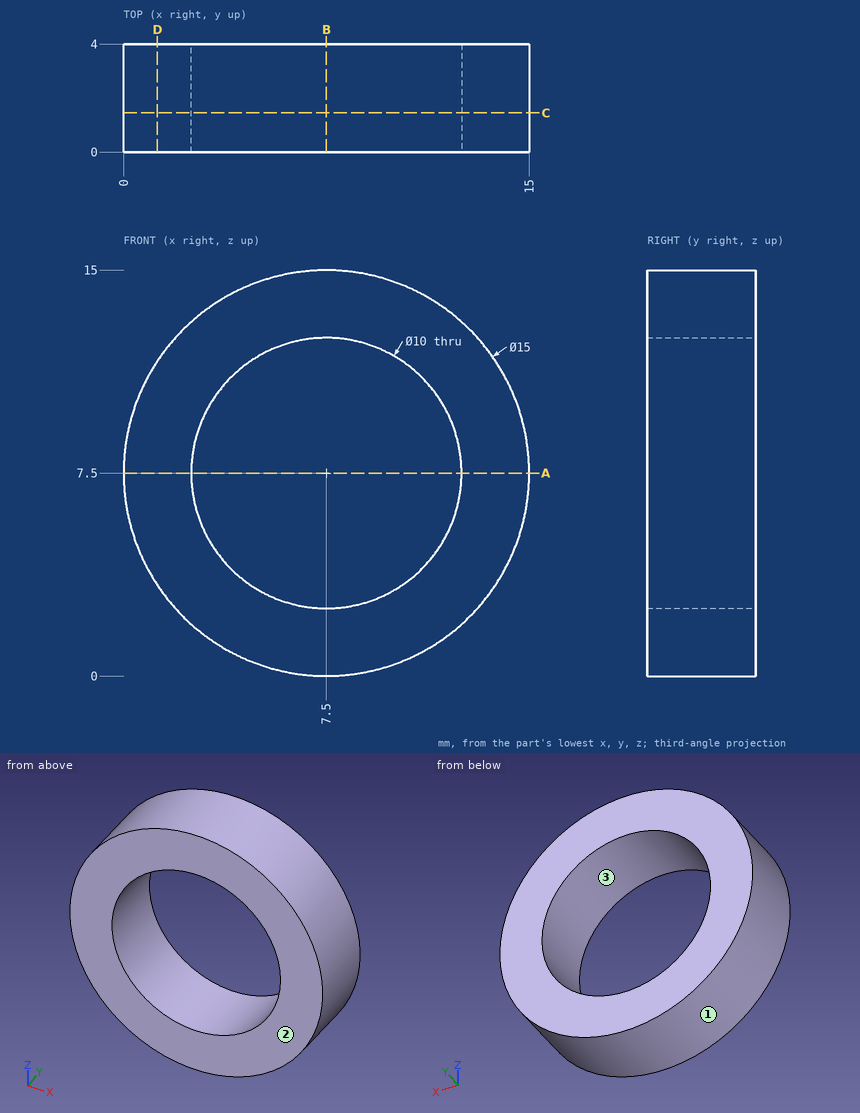
Input: dimensioned drawing with shaded views. Units: mm. Origin: part minimum x, y, z. Coordinates: 2 decimals unless noted, no trailing zeros. Loops run counter-clockwise (first coordinate to the right, second up) from the corner with the lowest first, then second, coordinate; pieces in that order, holes last. Notation, with made-up numbers: M 57,58.25 L 61,58.25 A31 ccw 61,94.25 Z; hole C 31.25,-1 d9. An arc over 180 degrees is marked long. Use a Markdown table: item, result. Add a question column.
Q1. Section query C-C, the plane y = 1.45. Return loops of the section in (x, z).
Q2. Section query A-A, the plane z = 7.5. Return loops of the section in (x, y), and give its area (3 significant figures).
Q3. Section query B-B, the plane x = 7.5. Return loops of the section in (y, z).
Q4. Draft query along Z for the marked faces 1, 2 and 3. Return one class per face: pulls with the +Z half, pulls with the -Z half, needs draft (parallel to the pull), parting line crosses it, or undercut.
Q5. First-contact query: pin 1 (1 mm diameter, centred on y = 2.5, z = 10, fed in from +X); pin 2 (1 mm diameter, centred on x = 3, y = 1, fed in from +Z). Flat tips, straight axial feed; report the tip coordinate or a pass-through.
Q6. Material intervals for L1, parallel to Z at x = 7.5, y = 3.05; L2, parallel to X at y = 3.7, z = 5, sorted ascending.
Q7. Section query D-D, the plane x = 1.25. Return loops of the section in (y, z).
Result:
| question | item | result |
|---|---|---|
| 1 | outline | C 7.5,7.5 d15; hole C 7.5,7.5 d10 |
| 2 | outline | M 0,0 L 2.5,0 L 2.5,4 L 0,4 Z; M 12.5,0 L 15,0 L 15,4 L 12.5,4 Z |
| 2 | area | 20.0 mm2 |
| 3 | outline | M 0,0 L 4,0 L 4,2.5 L 0,2.5 Z; M 0,12.5 L 4,12.5 L 4,15 L 0,15 Z |
| 4 | face 1 | parting line crosses it |
| 4 | face 2 | needs draft |
| 4 | face 3 | undercut |
| 5 | pin 1 | stops at x = 14.73 |
| 5 | pin 2 | stops at z = 13.84 |
| 6 | L1 | z = 0 to 2.5, 12.5 to 15 |
| 6 | L2 | x = 0.43 to 3.17, 11.83 to 14.57 |
| 7 | outline | M 0,3.35 L 4,3.35 L 4,11.65 L 0,11.65 Z |
